Geometry check sheet. Reference: the model listing, model coordinates, mm. A direction names the side the tool comes from. Coordinates: 2 decimals unless noted, no trailing zeros. Write each loop counter-clockwise with the first axis right and the second up, starting at its lowest first coordinate (ties: lowest second). Pieces come first, ordered by that corner, then holes. Notation, with made-up numbers: (-36.5, -31) -> (-28.5, -31) arc R29 ccw to (-28.5, -8) -> close; hole circle Ø2 at (29.25, 72.25). An arc over 180 degrees is marked (long way). Answer in a Markdown table with one row per item. Add a question column.
1. Set-up check for faces 5 (the cylindrical face through (-20.14, 7.37, 20.1)), 6 (the flat face through (17, 6.54, 17)), 7 (the flat face through (10.16, 12, -19)): record each of +Z, -Z, +X, -X, +Y, -Y from which the full face is reachable in a straight line by a thin tool's end or side.
2. Cross-section at B-B on x = -13. Record the cut outline in (y, z), and give its area (3 significant figures).
3. Scan lines: L1, parallel to Z at x = 8, y = 6.5; L2, parallel to X at y = 4, z = 0; L3, parallel to Z at x = -13.5, y = 7.5. Record each from-to range of solid material in increasing order. Write a range as from..to.
4. Cross-section at D-D on x = 8. Record the cut outline in (y, z).
5. Cross-section at A-A on y = -7. Record the cut outline in (x, z), and give its area (3 significant figures).
6. Cross-section at C-C on z = -9. Record the cut outline in (x, y).
7. Mould release check, pull along Y, two halves, no side actions. Record for faces 1 (the cylindrical face through (-0.294, -5.845, -0.423)), 2 (the flat face through (0, 14.54, 18)), 3 (the cylindrical face through (-19.05, 10.6, 16.91)), 4 (the flat face through (-0.294, -4.93, 6.725)): pulls with the +Y half, pulls with the -Y half, needs draft (parallel to the pull), parting line crosses it, or undercut.
8. Depth check by flat-ended pin: P1, Ø4.5, axis at x = -17, z = 17, coming from the -Y side; P2, Ø5, axis at x = -4, y = -8.5, coming from the -Z side; P3, Ø2.5, axis at x = -8, z = 0, coming from the +Y side. Enter the tip coordinate at first touch or a pass-through.
```python
from build123d import *

# Parameters (mm, degrees)
SKETCH1_W           = 42
SKETCH1_H           = 42
BOSS_EXTRUDE1_DEPTH = 2.54
SKETCH2_W           = 42
SKETCH2_H           = 42
BOSS_EXTRUDE2_DEPTH = 12
SKETCH4_R           = 3.25
BOSS_EXTRUDE4_DEPTH = 42
SKETCH9_R           = 6.25
SKETCH9_R_2         = 2.05
BOSS_EXTRUDE5_DEPTH = 6.5
SKETCH10_R          = 2.05
CUT_EXTRUDE1_DEPTH  = 8
SKETCH12_W          = 20.32
SKETCH12_H          = 5
CUT_EXTRUDE2_DEPTH  = 4
FILLET1_R           = 3


with BuildPart() as part:
    # Sketch1 → Boss-Extrude1 (new body)
    with BuildSketch(Plane(origin=(0, 0, 0), x_dir=(1, 0, 0), z_dir=(0, 1, 0))):
        Rectangle(SKETCH1_W, SKETCH1_H)
    extrude(amount=BOSS_EXTRUDE1_DEPTH)

    # Sketch2 → Boss-Extrude2 (add)
    with BuildSketch(Plane(origin=(0, 2.54, 0), x_dir=(1, 0, 0), z_dir=(0, 1, 0))):
        Rectangle(SKETCH2_W, SKETCH2_H)
        with BuildLine():
            Line((-17, 11.522774425), (-17, -11.522774425))
            ThreePointArc((-17, -11.522774425), (-16.869274473, -11.859874356), (-16.545454545, -12.020704023))
            ThreePointArc((-16.545454545, -12.020704023), (-13.464466094, -13.464466094), (-12.020704023, -16.545454545))
            ThreePointArc((-12.020704023, -16.545454545), (-11.859874356, -16.869274473), (-11.522774425, -17))
            Line((-11.522774425, -17), (11.522774425, -17))
            ThreePointArc((11.522774425, -17), (11.859874356, -16.869274473), (12.020704023, -16.545454545))
            ThreePointArc((12.020704023, -16.545454545), (13.464466094, -13.464466094), (16.545454545, -12.020704023))
            ThreePointArc((16.545454545, -12.020704023), (16.869274473, -11.859874356), (17, -11.522774425))
            Line((17, -11.522774425), (17, 11.522774425))
            ThreePointArc((17, 11.522774425), (16.869274473, 11.859874356), (16.545454545, 12.020704023))
            ThreePointArc((16.545454545, 12.020704023), (13.464466094, 13.464466094), (12.020704023, 16.545454545))
            ThreePointArc((12.020704023, 16.545454545), (11.859874356, 16.869274473), (11.522774425, 17))
            Line((11.522774425, 17), (-11.522774425, 17))
            ThreePointArc((-11.522774425, 17), (-11.859874356, 16.869274473), (-12.020704023, 16.545454545))
            ThreePointArc((-12.020704023, 16.545454545), (-13.464466094, 13.464466094), (-16.545454545, 12.020704023))
            ThreePointArc((-16.545454545, 12.020704023), (-16.869274473, 11.859874356), (-17, 11.522774425))
        make_face(mode=Mode.SUBTRACT)
    extrude(amount=BOSS_EXTRUDE2_DEPTH)

    # Sketch4 → Boss-Extrude4 (add)
    with BuildSketch(Plane.ZY.offset(21)):
        with BuildLine():
            Line((7.5, 0), (5.927131841, -10))
            ThreePointArc((5.927131841, -10), (0, -15.067740305), (-5.927131841, -10))
            Line((-5.927131841, -10), (-7.5, 0))
            Line((-7.5, 0), (7.5, 0))
        make_face()
        with Locations((0, -9.067740305)):
            Circle(SKETCH4_R, mode=Mode.SUBTRACT)
    extrude(amount=-BOSS_EXTRUDE4_DEPTH)

    # Sketch9 → Boss-Extrude5 (add)
    with BuildSketch(Plane(origin=(0, 2.54, 0), x_dir=(1, 0, 0), z_dir=(0, 1, 0))):
        with Locations((8, 0)):
            Circle(SKETCH9_R)
        with Locations((8, 0)):
            Circle(SKETCH9_R_2, mode=Mode.SUBTRACT)
        with Locations((-8, 0)):
            Circle(SKETCH9_R)
        with Locations((-8, 0)):
            Circle(SKETCH9_R_2, mode=Mode.SUBTRACT)
    extrude(amount=BOSS_EXTRUDE5_DEPTH)

    # Sketch10 → Cut-Extrude1 (cut)
    with BuildSketch(Plane(origin=(0, 14.54, 0), x_dir=(1, 0, 0), z_dir=(0, 1, 0))):
        with Locations((-17, 17)):
            Circle(SKETCH10_R)
        with Locations((17, 17)):
            Circle(SKETCH10_R)
        with Locations((-17, -17)):
            Circle(SKETCH10_R)
        with Locations((17, -17)):
            Circle(SKETCH10_R)
    extrude(amount=-CUT_EXTRUDE1_DEPTH, mode=Mode.SUBTRACT)

    # Sketch12 → Cut-Extrude2 (cut)
    with BuildSketch(Plane(origin=(0, 0, -21), x_dir=(-1, 0, 0), z_dir=(0, 0, -1))):
        with Locations((0, 12.04)):
            Rectangle(SKETCH12_W, SKETCH12_H)
    extrude(amount=-CUT_EXTRUDE2_DEPTH, mode=Mode.SUBTRACT)

    # Fillet1
    fillet1_edges = [part.edges().sort_by_distance(p)[0] for p in [
        (21, 7.27, 21),
        (-21, 7.27, 21),
        (-21, 7.27, -21),
        (21, 7.27, -21),
    ]]
    fillet(fillet1_edges, radius=FILLET1_R)


solid = part.part
```
Results found:
| question | item | result |
|---|---|---|
| 1 | face 5 | +Z, -X, +Y, -Y |
| 1 | face 6 | +Y |
| 1 | face 7 | -Z, +Y |
| 2 | outline | (-10, -5.93) -> (0, -7.5) -> (0, -21) -> (14.54, -21) -> (14.54, -14) -> (2.54, -14) -> (2.54, -3.75) -> (9.04, -3.75) -> (9.04, 3.75) -> (2.54, 3.75) -> (2.54, 14) -> (14.54, 14) -> (14.54, 21) -> (0, 21) -> (0, 7.5) -> (-10, 5.93) arc R6 ccw to start; hole circle Ø6.5 at (-9.07, 0) |
| 2 | area | 470 mm^2 |
| 3 | L1 | z = -21..-17, -6.25..-2.05, 2.05..6.25, 17..21 |
| 3 | L2 | x = -21..-17, -14.25..-10.05, -5.95..-1.75, 1.75..5.95, 10.05..14.25, 17..21 |
| 3 | L3 | z = -21..-13.43, -2.97..2.97, 13.43..21 |
| 4 | outline | (-10, -5.93) -> (0, -7.5) -> (0, -21) -> (9.54, -21) -> (9.54, -17) -> (2.54, -17) -> (2.54, -6.25) -> (9.04, -6.25) -> (9.04, -2.05) -> (2.54, -2.05) -> (2.54, 2.05) -> (9.04, 2.05) -> (9.04, 6.25) -> (2.54, 6.25) -> (2.54, 17) -> (14.54, 17) -> (14.54, 21) -> (0, 21) -> (0, 7.5) -> (-10, 5.93) arc R6 ccw to start; hole circle Ø6.5 at (-9.07, 0) |
| 5 | outline | (-21, -6.4) -> (21, -6.4) -> (21, -2.51) -> (-21, -2.51) -> close; (-21, 2.51) -> (21, 2.51) -> (21, 6.4) -> (-21, 6.4) -> close |
| 5 | area | 327 mm^2 |
| 6 | outline | (-21, 0) -> (21, 0) -> (21, 14.54) -> (17, 14.54) -> (17, 2.54) -> (-17, 2.54) -> (-17, 14.54) -> (-21, 14.54) -> close |
| 7 | face 1 | undercut |
| 7 | face 2 | pulls with the +Y half |
| 7 | face 3 | needs draft |
| 7 | face 4 | pulls with the -Y half |
| 8 | P1 | stops at y = 0 |
| 8 | P2 | stops at z = -6.56 |
| 8 | P3 | stops at y = 2.54 |
